Build history of the part. All positions in model axes, mm. Face numbers are marked on the shaded views. A direction names the side the tool comes from. Give positions to 0.01 mm unless a question says otherwise; leave off trailing zeros. Order: outer loops, then holes, each group sorted by start corner. A loop starts at its lowest first (then second) coordinate and runs counter-clockwise, first axis right, second up. Notation, with made-up numbers: (-35, -8) - (0, -8) arc R23 ccw to (0, 26) - close; hole circle Ø9 at (-10, -3.5). An arc over 180 degrees is marked (long way). Use a Markdown table: item, result. Add a question column.
(1) Slice it at C-C (z = 4.55). Write the cut outline in (x, y), then the cut area to 3 significant figures.
(2) Flat gauge pins, fed straight in: pin 1 (5 mm diameter, centred on y = 5.5, z = 26.5, fed in from +X); pin 2 (1.4 mm diameter, centred on x = 16, y = 2, fed in from +Z); pin 3 (5 mm diameter, centred on x = 20, y = -2.5, fed in from +Z). Where does each tip first touch, or does it go through?
(3) Slice it at B-B (y = 5.5). Write the cut outline in (x, z), then the cut area to 3 significant figures.
(4) Mould opens along X. For the marked faces 4, 5, 6 and 7 say: +X half, -X half, draft (parallel to the pull), parting line (faces both ways), or undercut.
(5) Which spindle directions (+Z, -Z, +X, -X, +Y, -Y) get a long thin tool onto all of the face, cutting with end or side? Do the marked faces 1, 2 and 3. Say none if no direction does.
(6) Wall check: line 1 (Y direction, x = 3, z = 28) (3 decimals); line 2 (Z direction, x = 6.5, y = 7.4); line 3 (X direction, y = 1.35, z = 4.55). Give the ranges that are in metal, low to high.
(7) Slice it at A-A (y = 3.5). Write the cut outline in (x, z).
(8) Slice it at D-D (x = 22). Write the cut outline in (y, z).
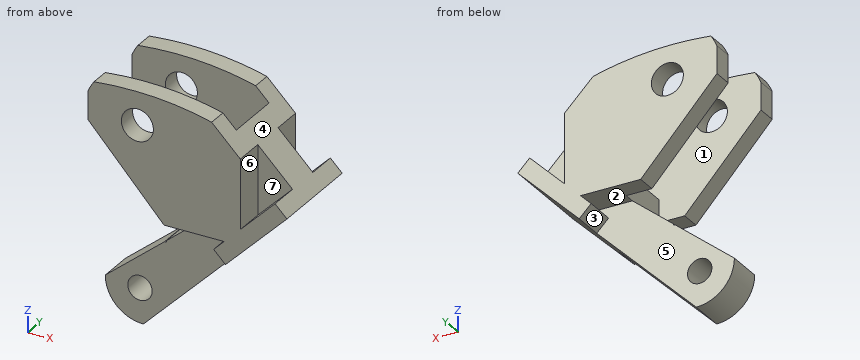
from build123d import *

# Parameters (mm, degrees)
SKETCH_1_R           = 1.6
EXTRUDE_1_DEPTH      = 4.65
SKETCH_7_W           = 9
SKETCH_7_H           = 19
EXTRUDE_4_DEPTH      = 4
SKETCH_8_W           = 9
SKETCH_8_H           = 19
EXTRUDE_5_DEPTH      = 4
SKETCH_9_W           = 16
SKETCH_9_H           = 7.5
CUT_EXTRUDE_3_DEPTH  = 9
SKETCH_11_R          = 2.1
CUT_EXTRUDE_5_DEPTH  = 26.4
EXTRUDE_6_DEPTH      = 9
SKETCH_13_W          = 19
SKETCH_13_H          = 12.65
EXTRUDE_7_DEPTH      = 2
SKETCH_15_W          = 7.596607022
SKETCH_15_H          = 7.5
CUT_EXTRUDE_6_DEPTH  = 8
CUT_EXTRUDE_7_DEPTH  = 8
EXTRUDE_8_DEPTH      = 4.65
CUT_EXTRUDE_9_DEPTH  = 4.65
SKETCH_20_W          = 5.380169682
SKETCH_20_H          = 3
CUT_EXTRUDE_10_DEPTH = 7.5
CUT_EXTRUDE_11_DEPTH = 4.65
CUT_EXTRUDE_13_DEPTH = 13
CUT_EXTRUDE_15_DEPTH = 13
SKETCH_26_W          = 18.396488504
SKETCH_26_H          = 12.65
EXTRUDE_9_DEPTH      = 2.2
SKETCH_28_W          = 2.5
SKETCH_28_H          = 12.65
CUT_EXTRUDE_17_DEPTH = 18
CUT_EXTRUDE_18_DEPTH = 14
SKETCH_31_W          = 5
SKETCH_31_H          = 12.65
CUT_EXTRUDE_19_DEPTH = 20


with BuildPart() as part:
    # 草图1 → 凸台-拉伸1 (new body)
    with BuildSketch(Plane(origin=(0, 0, 0), x_dir=(1, 0, 0), z_dir=(0, 1, 0))):
        with BuildLine():
            Line((5, 0), (20, 0))
            Line((20, 0), (20, -16))
            Line((20, -16), (9, -16))
            Line((9, -16), (9, -35))
            Line((9, -35), (0, -35))
            Line((0, -35), (0, -27))
            Line((0, -27), (0, -5))
            ThreePointArc((0, -5), (1.464466094, -1.464466094), (5, 0))
        make_face()
        with Locations((4.55, -4.55)):
            Circle(SKETCH_1_R, mode=Mode.SUBTRACT)
    extrude(amount=EXTRUDE_1_DEPTH)

    # 草图7 → 凸台-拉伸4 (add)
    with BuildSketch(Plane(origin=(0, 4.65, 0), x_dir=(1, 0, 0), z_dir=(0, 1, 0))):
        with Locations((4.5, -25.5)):
            Rectangle(SKETCH_7_W, SKETCH_7_H)
    extrude(amount=EXTRUDE_4_DEPTH)

    # 草图8 → 凸台-拉伸5 (add)
    with BuildSketch(Plane.XZ):
        with Locations((4.5, 25.5)):
            Rectangle(SKETCH_8_W, SKETCH_8_H)
    extrude(amount=EXTRUDE_5_DEPTH)

    # 草图9 → 切除-拉伸3 (cut)
    with BuildSketch(Plane.ZY):
        with Locations((27, 2.325)):
            Rectangle(SKETCH_9_W, SKETCH_9_H)
    extrude(amount=-CUT_EXTRUDE_3_DEPTH, mode=Mode.SUBTRACT)

    # 草图11 → 切除-拉伸5 (cut)
    with BuildSketch(Plane(origin=(0, 8.65, 0), x_dir=(1, 0, 0), z_dir=(0, 1, 0))):
        with Locations((6.5, -28)):
            Circle(SKETCH_11_R)
    extrude(amount=-CUT_EXTRUDE_5_DEPTH, mode=Mode.SUBTRACT)

    # 草图12 → 凸台-拉伸6 (add)
    with BuildSketch(Plane(origin=(9, 0, 0), x_dir=(0, 0, -1), z_dir=(1, 0, 0))):
        Polygon((-35, 8.65), (-35, 6.075), (-19, 6.075), (-19, -1.425), (-35, -1.425), (-35, -4), (-16, -4), (-16, 8.65), align=None)
    extrude(amount=EXTRUDE_6_DEPTH)

    # 草图13 → 凸台-拉伸7 (add)
    with BuildSketch(Plane(origin=(18, 0, 0), x_dir=(0, 0, -1), z_dir=(1, 0, 0))):
        with Locations((-25.5, 2.325)):
            Rectangle(SKETCH_13_W, SKETCH_13_H)
    extrude(amount=EXTRUDE_7_DEPTH)

    # 草图15 → 切除-拉伸6 (cut)
    with BuildSketch(Plane.ZY):
        with Locations((15.201696489, 2.325)):
            Rectangle(SKETCH_15_W, SKETCH_15_H)
    extrude(amount=-CUT_EXTRUDE_6_DEPTH, mode=Mode.SUBTRACT)

    # 草图16 → 切除-拉伸7 (cut)
    with BuildSketch(Plane(origin=(0, 4.65, 0), x_dir=(1, 0, 0), z_dir=(0, 1, 0))):
        Polygon((0, -5), (5.890898071, -11.403392978), (0, -11.403392978), align=None)
    extrude(amount=-CUT_EXTRUDE_7_DEPTH, mode=Mode.SUBTRACT)

    # 草图17 → 凸台-拉伸8 (add)
    with BuildSketch(Plane.XZ):
        with BuildLine():
            Line((20, 35), (20, 15))
            Line((20, 15), (31.064630957, 26.064630957))
            ThreePointArc((31.064630957, 26.064630957), (26.002686727, 31.114774273), (20, 35))
        make_face()
    extrude(amount=-EXTRUDE_8_DEPTH)

    # 草图19 → 切除-拉伸9 (cut)
    with BuildSketch(Plane(origin=(0, 4.65, 0), x_dir=(1, 0, 0), z_dir=(0, 1, 0))):
        Polygon((20, -15), (5, 0), (20, 0), align=None)
    extrude(amount=-CUT_EXTRUDE_9_DEPTH, mode=Mode.SUBTRACT)

    # 草图20 → 切除-拉伸10 (cut)
    with BuildSketch(Plane(origin=(0, -1.425, 0), x_dir=(1, 0, 0), z_dir=(0, 1, 0))):
        with Locations((10.690084841, -17.5)):
            Rectangle(SKETCH_20_W, SKETCH_20_H)
    extrude(amount=CUT_EXTRUDE_10_DEPTH, mode=Mode.SUBTRACT)

    # 草图21 → 切除-拉伸11 (cut)
    with BuildSketch(Plane.XZ):
        Polygon((13.380169682, 16), (0, 5), (8, 16), align=None)
    extrude(amount=-CUT_EXTRUDE_11_DEPTH, mode=Mode.SUBTRACT)

    # 草图22 → 切除-拉伸13 (cut)
    with BuildSketch(Plane(origin=(0, 8.65, 0), x_dir=(1, 0, 0), z_dir=(0, 1, 0))):
        Polygon((0, -16), (10, -16), (0, -27), align=None)
    extrude(amount=-CUT_EXTRUDE_13_DEPTH, mode=Mode.SUBTRACT)

    # 草图23 → 切除-拉伸15 (cut)
    with BuildSketch(Plane(origin=(0, 8.65, 0), x_dir=(1, 0, 0), z_dir=(0, 1, 0))):
        with BuildLine():
            Line((6.5, -35), (0, -35))
            Line((0, -35), (0, -30.598076211))
            ThreePointArc((0, -30.598076211), (2.574858823, -33.79596987), (6.5, -35))
        make_face()
    extrude(amount=-CUT_EXTRUDE_15_DEPTH, mode=Mode.SUBTRACT)

    # 草图26 → 凸台-拉伸9 (add)
    with BuildSketch(Plane(origin=(2.5, 0, -2.5), x_dir=(-0.707106781, 0, -0.707106781), z_dir=(0.707106781, 0, -0.707106781))):
        with Locations((-31.198244252, 2.325)):
            Rectangle(SKETCH_26_W, SKETCH_26_H)
    extrude(amount=-EXTRUDE_9_DEPTH)

    # 草图28 → 切除-拉伸17 (cut)
    with BuildSketch(Plane(origin=(2.5, 0, -2.5), x_dir=(-0.707106781, 0, -0.707106781), z_dir=(0.707106781, 0, -0.707106781))):
        with Locations((-39.646488504, 2.325)):
            Rectangle(SKETCH_28_W, SKETCH_28_H)
    extrude(amount=-CUT_EXTRUDE_17_DEPTH, mode=Mode.SUBTRACT)

    # 草图29 → 切除-拉伸18 (cut)
    with BuildSketch(Plane.XZ.offset(4)):
        with BuildLine():
            Line((29.650417395, 24.650417395), (19.300834789, 35))
            Line((19.300834789, 35), (1.773611639, 35))
            Line((1.773611639, 35), (0.803925841, 32.06875155))
            add(Edge.make_bspline(
                [(29.650417395, 24.650417395), (16.711479186, 33.756910479), (0.803925841, 32.06875155)],
                knots=[0, 0, 0, 1, 1, 1], degree=2))
        make_face()
    extrude(amount=-CUT_EXTRUDE_18_DEPTH, mode=Mode.SUBTRACT)

    # 草图31 → 切除-拉伸19 (cut)
    with BuildSketch(Plane(origin=(2.5, 0, -2.5), x_dir=(-0.707106781, 0, -0.707106781), z_dir=(0.707106781, 0, -0.707106781))):
        with Locations((-35.896488504, 2.325)):
            Rectangle(SKETCH_31_W, SKETCH_31_H)
    extrude(amount=-CUT_EXTRUDE_19_DEPTH, mode=Mode.SUBTRACT)


solid = part.part
Solution:
| question | item | result |
|---|---|---|
| 1 | outline | (0.02, 0) - (2.95, 0) - (2.95, 4.65) - (0.02, 4.65) - close; (6.15, 0) - (9.55, 0) - (9.55, 4.65) - (6.15, 4.65) - close |
| 1 | area | 29.4 mm2 |
| 2 | pin 1 | x = 23.08 |
| 2 | pin 2 | z = 19 |
| 2 | pin 3 | z = 29.73 |
| 3 | outline | (13.38, 16) - (17.89, 16) - (16.5, 14.61) - (18.06, 13.06) - (26.11, 21.11) - (24.56, 22.67) - (20, 18.11) - (20, 27.23) - (18, 29.23) - (18, 19) - (13.38, 19) - close |
| 3 | area | 61.2 mm2 |
| 4 | face 4 | +X half |
| 4 | face 5 | draft |
| 4 | face 6 | undercut |
| 4 | face 7 | undercut |
| 5 | face 1 | +Z, -X |
| 5 | face 2 | -X, +Y |
| 5 | face 3 | -Z, -X, +Y |
| 6 | line 1 | -4 to -1.425, 6.075 to 8.65 |
| 6 | line 2 | 19.85 to 25.9, 30.1 to 32.33 |
| 6 | line 3 | 0.02 to 2.95, 6.15 to 9.55 |
| 7 | outline | (0, 5) arc R5 ccw to (5, 0) - (26.11, 21.11) - (18, 29.23) - (18, 19) - (13.38, 19) - (13.38, 16) - (8, 11.58) - (8, 11.4) - (7.79, 11.4) - close; hole circle Ø3.2 at (4.55, 4.55) |
| 8 | outline | (-4, 17) - (8.65, 17) - (8.65, 20.11) - (4.65, 20.11) - (4.65, 25.23) - (0, 25.23) - (0, 20.11) - (-4, 20.11) - close |
